Geometry: final body of the model. Coordinates: model frame, mm. Give positions to 0.01 mm unless a question says otherwise; leave off trailing zeros. Write each loop counter-clockwise with the first axis right and the second up, starting at its lowest first coordinate (ties: lowest second). Pieces come first, ordered by that corner, then holes. Notation, with made-up numbers: M 30,38.5 L 37,38.5 A20 ccw 37,47.5 Z; hole C 66.25,-24.75 d1. An arc over 180 degrees is marked long. One line per question, with ' | ' between items.
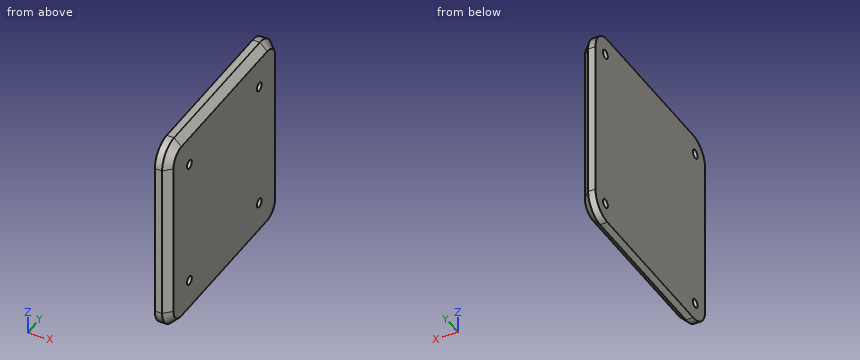
Autodesk Inventor part; units mm, degrees
ref_plane "YZ Plane" through (0, 0, 0) normal (1, 0, 0) x (0, 1, 0)
ref_plane "XZ Plane" through (0, 0, 0) normal (0, 1, 0) x (-1, 0, 0)
ref_plane "XY Plane" through (0, 0, 0) normal (0, 0, 1) x (1, 0, 0)
sketch "草圖1" plane through (0, 0, 0) normal (1, 0, 0) x (0, 1, 0)
  line L0 (-137.5, 137.5) -> (137.5, 137.5)
  line L1 (137.5, 137.5) -> (137.5, -137.5)
  line L2 (137.5, -137.5) -> (-137.5, -137.5)
  line L3 (-137.5, -137.5) -> (-137.5, 137.5)
  line L4 (-137.5, 137.5) -> (137.5, -137.5) construction
  line L5 (137.5, 137.5) -> (-137.5, -137.5) construction
  point P0 (0, 0)
  dimension "d0" = 275
  dimension "d1" = 275
extrude "擠出1" add sketch "草圖1" along normal blind 20
fillet "圓角1" radius 30 4 edges at (10, 137.5, 137.5) (10, -137.5, 137.5) (10, 137.5, -137.5) (10, -137.5, -137.5)
chamfer "倒角1" distance 10 angle 45 8 edges at (20, 0, 137.5) (20, -128.7132, 128.7132) (20, -137.5, 0) (20, -128.7132, -128.7132) (20, 0, -137.5) (20, 128.7132, -128.7132) (20, 137.5, 0) (20, 128.7132, 128.7132)
sketch "草圖2" plane through (20, 0, 0) normal (1, 0, 0) x (0, 0, -1)
  line L0 (-87.5, -87.5) -> (87.5, -87.5)
  line L1 (87.5, -87.5) -> (87.5, 87.5)
  line L2 (87.5, 87.5) -> (-87.5, 87.5)
  line L3 (-87.5, 87.5) -> (-87.5, -87.5)
  line L4 (-87.5, -87.5) -> (87.5, 87.5) construction
  line L5 (87.5, -87.5) -> (-87.5, 87.5) construction
  point P0 (0, 0)
  dimension "d8" = 175
  dimension "d9" = 175
hole "孔1" at (20, 87.5, 87.5) at (20, 87.5, -87.5) at (20, -87.5, 87.5) at (20, -87.5, -87.5) direction (-1, 0, 0) diameter 12 depth 10 tip angle 118
sketch "草圖3" plane through (0, 0, 0) normal (-1, 0, 0) x (0, 0, 1)
  arc A0 (-137.5, -107.5) -> (-107.5, -137.5) centre (-107.5, -107.5) ccw
  line L0 (-107.5, -137.5) -> (107.5, -137.5)
  arc A1 (107.5, -137.5) -> (137.5, -107.5) centre (107.5, -107.5) ccw
  line L1 (137.5, -107.5) -> (137.5, 107.5)
  arc A2 (137.5, 107.5) -> (107.5, 137.5) centre (107.5, 107.5) ccw
  line L2 (107.5, 137.5) -> (-107.5, 137.5)
  arc A3 (-107.5, 137.5) -> (-137.5, 107.5) centre (-107.5, 107.5) ccw
  line L3 (-137.5, 107.5) -> (-137.5, -107.5)
  line L4 (112.5, 112.5) -> (-112.5, 112.5)
  line L5 (-112.5, 112.5) -> (-112.5, -112.5)
  line L6 (-112.5, -112.5) -> (112.5, -112.5)
  line L7 (112.5, -112.5) -> (112.5, 112.5)
  line L8 (112.5, 112.5) -> (-112.5, -112.5) construction
  line L9 (-112.5, 112.5) -> (112.5, -112.5) construction
  point P0 (0, 0)
  dimension "d17" = 225
  dimension "d18" = 225
hole "孔2" at (0, -112.5, 112.5) at (0, -112.5, -112.5) at (0, 112.5, -112.5) at (0, 112.5, 112.5) direction (1, 0, 0) diameter 12 depth 10 tip angle 118
properties part number "exercise3-1-2"
(1) First-contact query: P1, Ø6, axis at x = 15, y = -29.5, coming from the +Z side; P2, Ø1, axis at x = 11, z = 92, coming from the +Y side. Flat tips, straight axial feed; report the tip coordinate or a pass-through.
Working result:
P1: stops at z = 135.5 | P2: stops at y = 137
(2) Material intervals for L1, parallel to Z at x = 17.75, y = -87.5; L2, parallel to Z at x = 3, y = -112.5; L3, parallel to Y at x = 10.5, z = 92.5, sorted ascending. Write a range as [from, to].
Working result:
L1: z = [-129.75, -93.5], [-81.5, 81.5], [93.5, 129.75] | L2: z = [-137.08, -118.5], [-106.5, 106.5], [118.5, 137.08] | L3: y = [-137, -90.82], [-84.18, 84.18], [90.82, 137]
(3) Cut plane A-A, the plane z = 29. Return loops of the section in (x, y).
Working result:
outline: M 0,-137.5 L 10,-137.5 L 20,-127.5 L 20,127.5 L 10,137.5 L 0,137.5 Z
